from build123d import *

# Parameters (mm, degrees)
SKETCH1_W           = 126
SKETCH1_H           = 150
SKETCH1_W_2         = 112
SKETCH1_H_2         = 136
BOSS_EXTRUDE1_DEPTH = 7
SKETCH2_R           = 2.05
CUT_EXTRUDE1_DEPTH  = 6
SKETCH3_R           = 1.35
CUT_EXTRUDE2_DEPTH  = 8
SKETCH4_R           = 2.5
CUT_EXTRUDE3_DEPTH  = 3
SKETCH5_R           = 1.35
CUT_EXTRUDE4_DEPTH  = 8
SKETCH6_R           = 2.5
CUT_EXTRUDE5_DEPTH  = 3
CUT_EXTRUDE6_DEPTH  = 0.2
SKETCH8_W           = 2.7
SKETCH8_H           = 2.7
CUT_EXTRUDE7_DEPTH  = 0.2
SKETCH9_R           = 2.05
CUT_EXTRUDE8_DEPTH  = 8
SKETCH10_W          = 6
SKETCH10_H          = 6
BOSS_EXTRUDE2_DEPTH = 4
SKETCH11_R          = 1.65
CUT_EXTRUDE9_DEPTH  = 5
CHAMFER1_SIZE       = 0.4


with BuildPart() as part:
    # Sketch1 → Boss-Extrude1 (new body)
    with BuildSketch(Plane.XY):
        Rectangle(SKETCH1_W, SKETCH1_H)
        Rectangle(SKETCH1_W_2, SKETCH1_H_2, mode=Mode.SUBTRACT)
    extrude(amount=BOSS_EXTRUDE1_DEPTH)

    # Sketch2 → Cut-Extrude1 (cut)
    with BuildSketch(Plane(origin=(63, 0, 0), x_dir=(0, 0, -1), z_dir=(1, 0, 0))):
        with Locations((-3.5, 71.5)):
            Circle(SKETCH2_R)
        with Locations((-3.5, -71.5)):
            Circle(SKETCH2_R)
        with Locations((-3.5, 35.5)):
            Circle(SKETCH2_R)
        with Locations((-3.5, -26.5)):
            Circle(SKETCH2_R)
    cut_extrude1 = extrude(amount=-CUT_EXTRUDE1_DEPTH, mode=Mode.SUBTRACT)

    # Mirror1: Cut-Extrude1 across plane
    add(cut_extrude1.mirror(Plane(origin=(0, 0, 0), x_dir=(0, 0, 1), z_dir=(1, 0, 0))), mode=Mode.SUBTRACT)

    # Sketch3 → Cut-Extrude2 (cut, through all)
    with BuildSketch(Plane(origin=(0, -68, 0), x_dir=(1, 0, 0), z_dir=(0, 1, 0))):
        with Locations((-40, -3.5)):
            Circle(SKETCH3_R)
        with Locations((40, -3.5)):
            Circle(SKETCH3_R)
    extrude(amount=-CUT_EXTRUDE2_DEPTH, mode=Mode.SUBTRACT)

    # Sketch4 → Cut-Extrude3 (cut)
    with BuildSketch(Plane(origin=(0, -68, 0), x_dir=(1, 0, 0), z_dir=(0, 1, 0))):
        with Locations((-40, -3.5)):
            Circle(SKETCH4_R)
        with Locations((40, -3.5)):
            Circle(SKETCH4_R)
    extrude(amount=-CUT_EXTRUDE3_DEPTH, mode=Mode.SUBTRACT)

    # Sketch5 → Cut-Extrude4 (cut, through all)
    with BuildSketch(Plane.XY.offset(7)):
        with Locations((-59.5, 2)):
            Circle(SKETCH5_R)
        with Locations((59.5, 2)):
            Circle(SKETCH5_R)
        with Locations((-59.5, -35.5)):
            Circle(SKETCH5_R)
        with Locations((59.5, -35.5)):
            Circle(SKETCH5_R)
    extrude(amount=-CUT_EXTRUDE4_DEPTH, mode=Mode.SUBTRACT)

    # Sketch6 → Cut-Extrude5 (cut)
    with BuildSketch(Plane.XY.offset(7)):
        with Locations((-59.5, 2)):
            Circle(SKETCH6_R)
        with Locations((59.5, 2)):
            Circle(SKETCH6_R)
        with Locations((-59.5, -35.5)):
            Circle(SKETCH6_R)
        with Locations((59.5, -35.5)):
            Circle(SKETCH6_R)
    extrude(amount=-CUT_EXTRUDE5_DEPTH, mode=Mode.SUBTRACT)

    # Sketch7 → Cut-Extrude6 (cut)
    with BuildSketch(Plane.XY.offset(4)):
        with BuildLine():
            Line((-60.85, -0.104162541), (-60.85, 4.104162541))
            ThreePointArc((-60.85, 4.104162541), (-59.5, 4.5), (-58.15, 4.104162541))
            Line((-58.15, 4.104162541), (-58.15, -0.104162541))
            ThreePointArc((-58.15, -0.104162541), (-59.5, -0.5), (-60.85, -0.104162541))
        make_face()
        with BuildLine():
            Line((-60.85, -37.604162541), (-60.85, -33.395837459))
            ThreePointArc((-60.85, -33.395837459), (-59.5, -33), (-58.15, -33.395837459))
            Line((-58.15, -33.395837459), (-58.15, -37.604162541))
            ThreePointArc((-58.15, -37.604162541), (-59.5, -38), (-60.85, -37.604162541))
        make_face()
    cut_extrude6 = extrude(amount=-CUT_EXTRUDE6_DEPTH, mode=Mode.SUBTRACT)

    # Sketch8 → Cut-Extrude7 (cut)
    with BuildSketch(Plane.XY.offset(3.8)):
        with Locations((-59.5, -35.5)):
            Rectangle(SKETCH8_W, SKETCH8_H)
        with Locations((-59.5, 2)):
            Rectangle(SKETCH8_W, SKETCH8_H)
    cut_extrude7 = extrude(amount=-CUT_EXTRUDE7_DEPTH, mode=Mode.SUBTRACT)

    # Mirror2: Cut-Extrude6, Cut-Extrude7 across plane
    add(cut_extrude6.mirror(Plane(origin=(0, 0, 0), x_dir=(0, 0, 1), z_dir=(1, 0, 0))), mode=Mode.SUBTRACT)
    add(cut_extrude7.mirror(Plane(origin=(0, 0, 0), x_dir=(0, 0, 1), z_dir=(1, 0, 0))), mode=Mode.SUBTRACT)

    # Sketch9 → Cut-Extrude8 (cut, through all)
    with BuildSketch(Plane.XY.offset(7)):
        with Locations((-59.5, 65)):
            Circle(SKETCH9_R)
        with Locations((-59.5, -10)):
            Circle(SKETCH9_R)
    cut_extrude8 = extrude(amount=-CUT_EXTRUDE8_DEPTH, mode=Mode.SUBTRACT)

    # Mirror3: Cut-Extrude8 across plane
    add(cut_extrude8.mirror(Plane(origin=(0, 0, 0), x_dir=(0, 0, 1), z_dir=(1, 0, 0))), mode=Mode.SUBTRACT)

    # Sketch10 → Boss-Extrude2 (add)
    with BuildSketch(Plane(origin=(0, 0, 0), x_dir=(-1, 0, 0), z_dir=(0, 0, -1))):
        with Locations((53, -65)):
            Rectangle(SKETCH10_W, SKETCH10_H)
        with Locations((53, -35.5)):
            Rectangle(SKETCH10_W, SKETCH10_H)
    boss_extrude2 = extrude(amount=-BOSS_EXTRUDE2_DEPTH)

    # Sketch11 → Cut-Extrude9 (cut, through all)
    with BuildSketch(Plane.XY.offset(4)):
        with Locations((-53, -65)):
            Circle(SKETCH11_R)
        with Locations((-53, -35.5)):
            Circle(SKETCH11_R)
    cut_extrude9 = extrude(amount=-CUT_EXTRUDE9_DEPTH, mode=Mode.SUBTRACT)

    # Mirror4: Boss-Extrude2, Cut-Extrude9 across plane
    add(boss_extrude2.mirror(Plane(origin=(0, 0, 0), x_dir=(0, 0, 1), z_dir=(1, 0, 0))))
    add(cut_extrude9.mirror(Plane(origin=(0, 0, 0), x_dir=(0, 0, 1), z_dir=(1, 0, 0))), mode=Mode.SUBTRACT)

    # Chamfer1
    chamfer1_edges = [part.edges().sort_by_distance(p)[0] for p in [
        (56, 0, 7),
        (0, 68, 7),
        (-56, 0, 7),
        (0, -68, 7),
    ]]
    chamfer(chamfer1_edges, length=CHAMFER1_SIZE)


solid = part.part
Read the model definition and answer for the solid it produces. Units are mm, in the model's axes. A direction names the side the tool comes from. Coordinates: 2 decimals unless noted, no trailing zeros. Loops run counter-clockwise (first coordinate to the right, second up) from the corner with the lowest first, then second, coordinate; pieces in that order, holes last. Notation, with made-up numbers: (46, 63.5) -> (50, 63.5) arc R22 ccw to (50, 69.5) -> close; hole circle Ø2 at (2, 14.5). An arc over 180 degrees is marked (long way). Answer in a Markdown table with one row per item.
Item 1: For faces 4 (the cylindrical face through (-60.042, -69.467, 3.767)), 5 (the flat face through (-53, -32.5, 2)), 6 (the cylindrical face through (42.31, -69.48, 4.46)), determine the directions among +Z, -Z, +X, -X, +Y, -Y from which every point of the face is accessible in a straight line to the end or side of a thin tool.
Returned:
| item | result |
|---|---|
| face 4 | -X |
| face 5 | +Z, -Z |
| face 6 | none |
Item 2: For a pull along Y with two mould halves and no side action, classify faces 1 (the flat face through (-56.3, -5.2, 0)), 2 (the flat face through (-1, 75, 3)), 3 (the cylindrical face through (-60.042, 73.533, 3.767)) as released by +Y, released by -Y, zero draft, split by the parting line, or undercut.
Returned:
| item | result |
|---|---|
| face 1 | zero draft |
| face 2 | released by +Y |
| face 3 | undercut |
Item 3: A cutting plane is placed at C-C on y = -65. Determine the outline of the cut face in (x, z).
Returned:
| item | result |
|---|---|
| outline | (-63, 0) -> (-54.65, 0) -> (-54.65, 4) -> (-56, 4) -> (-56, 6.6) -> (-56.4, 7) -> (-63, 7) -> close; (-51.35, 0) -> (-50, 0) -> (-50, 4) -> (-51.35, 4) -> close; (50, 0) -> (51.35, 0) -> (51.35, 4) -> (50, 4) -> close; (54.65, 0) -> (63, 0) -> (63, 7) -> (56.4, 7) -> (56, 6.6) -> (56, 4) -> (54.65, 4) -> close |
Item 4: Each of these flat-tipped pins is pushed along its axis until it touches: P1, Ø5, axis at x = 52, y = -35.5, coming from the +Z side; P2, Ø2, axis at x = 53, y = -35.5, coming from the +Z side; P3, Ø0.6, axis at x = -60, y = 0.5, coming from the +Z side. Where does it stop, or does it pass through?
Returned:
| item | result |
|---|---|
| P1 | stops at z = 4 |
| P2 | passes through |
| P3 | stops at z = 3.8 |
Item 5: Straight lines are drawn through the part: line 1 along X through (y, z) = (2, 6.05); line 2 along X through (y, z) = (-67, 6.5); line 3 along Y through (x, z) = (-34, 6.5). For each, find the intervals that lie inside material, in ascending order. Write a range as [from, to].
Returned:
| item | result |
|---|---|
| line 1 | x = [-63, -62], [-57, -56], [56, 57], [62, 63] |
| line 2 | x = [-63, -56], [56, 63] |
| line 3 | y = [-75, -68], [68, 75] |
Item 6: A cutting plane is placed at D-D on x = 53. Determine the outline of the cut face in (y, z), plus the area to 3 significant figures.
Returned:
| item | result |
|---|---|
| outline | (-75, 0) -> (-66.65, 0) -> (-66.65, 4) -> (-68, 4) -> (-68, 6.6) -> (-68.4, 7) -> (-75, 7) -> close; (-63.35, 0) -> (-62, 0) -> (-62, 4) -> (-63.35, 4) -> close; (-38.5, 0) -> (-37.15, 0) -> (-37.15, 4) -> (-38.5, 4) -> close; (-33.85, 0) -> (-32.5, 0) -> (-32.5, 4) -> (-33.85, 4) -> close; (68, 0) -> (75, 0) -> (75, 7) -> (68.4, 7) -> (68, 6.6) -> close |
| area | 119 mm^2 |
Item 7: A cutting plane is placed at A-A on y = 35.5. Determine the outline of the cut face in (x, z), plus the area to 3 significant figures.
Returned:
| item | result |
|---|---|
| outline | (-63, 0) -> (-56, 0) -> (-56, 6.6) -> (-56.4, 7) -> (-63, 7) -> (-63, 5.55) -> (-57, 5.55) -> (-57, 1.45) -> (-63, 1.45) -> close; (56, 0) -> (63, 0) -> (63, 1.45) -> (57, 1.45) -> (57, 5.55) -> (63, 5.55) -> (63, 7) -> (56.4, 7) -> (56, 6.6) -> close |
| area | 48.6 mm^2 |
Item 8: A cutting plane is placed at B-B on x = 21. Determine the outline of the cut face in (y, z).
Returned:
| item | result |
|---|---|
| outline | (-75, 0) -> (-68, 0) -> (-68, 6.6) -> (-68.4, 7) -> (-75, 7) -> close; (68, 0) -> (75, 0) -> (75, 7) -> (68.4, 7) -> (68, 6.6) -> close |
